```python
from build123d import *

# Parameters (mm, degrees)
BOSS_EXTRUDE2_DEPTH  = 11.1125
SKETCH1_11_W         = 50.8
SKETCH1_11_H         = 50.8
BOSS_EXTRUDE3_DEPTH  = 609.6
SKETCH1_12_W         = 50.8
SKETCH1_12_H         = 50.8
BOSS_EXTRUDE4_DEPTH  = 609.6
SKETCH1_13_W         = 50.8
SKETCH1_13_H         = 50.8
BOSS_EXTRUDE5_DEPTH  = 609.6
SKETCH1_14_W         = 50.8
SKETCH1_14_H         = 50.8
BOSS_EXTRUDE6_DEPTH  = 609.6
SKETCH4_R            = 50.8
CUT_EXTRUDE2_DEPTH   = 12.1125
SKETCH5_W            = 165.1
SKETCH5_H            = 152.4
SKETCH5_W_2          = 139.7
SKETCH5_H_2          = 127
BOSS_EXTRUDE8_DEPTH  = 17.78
SKETCH13_W           = 50.8
SKETCH13_H           = 50.8
BOSS_EXTRUDE9_DEPTH  = 381
SKETCH14_R           = 55
SKETCH14_R_2         = 50.90263009
BOSS_EXTRUDE10_DEPTH = 284.5


with BuildPart() as part:
    # Sketch1 → Boss-Extrude2 (new body)
    with BuildSketch(Plane(origin=(0, 0, 0), x_dir=(1, 0, 0), z_dir=(0, 1, 0))):
        Polygon((-136.525, 152.4), (-187.325, 152.4), (-187.325, -203.2), (187.325, -203.2), (187.325, 203.2), (-136.525, 203.2), align=None)
    extrude(amount=BOSS_EXTRUDE2_DEPTH)

    # Sketch1<11> → Boss-Extrude3 (add)
    with BuildSketch(Plane(origin=(0, 0, 0), x_dir=(1, 0, 0), z_dir=(0, 1, 0))):
        with Locations((-161.925, 177.8)):
            Rectangle(SKETCH1_11_W, SKETCH1_11_H)
    extrude(amount=BOSS_EXTRUDE3_DEPTH)

    # Sketch1<12> → Boss-Extrude4 (add)
    with BuildSketch(Plane(origin=(0, 0, 0), x_dir=(1, 0, 0), z_dir=(0, 1, 0))):
        with Locations((-161.925, -177.8)):
            Rectangle(SKETCH1_12_W, SKETCH1_12_H)
    extrude(amount=BOSS_EXTRUDE4_DEPTH)

    # Sketch1<13> → Boss-Extrude5 (add)
    with BuildSketch(Plane(origin=(0, 0, 0), x_dir=(1, 0, 0), z_dir=(0, 1, 0))):
        with Locations((161.925, 177.8)):
            Rectangle(SKETCH1_13_W, SKETCH1_13_H)
    extrude(amount=BOSS_EXTRUDE5_DEPTH)

    # Sketch1<14> → Boss-Extrude6 (add)
    with BuildSketch(Plane(origin=(0, 0, 0), x_dir=(1, 0, 0), z_dir=(0, 1, 0))):
        with Locations((161.925, -177.8)):
            Rectangle(SKETCH1_14_W, SKETCH1_14_H)
    extrude(amount=BOSS_EXTRUDE6_DEPTH)

    # Sketch4 → Cut-Extrude2 (cut, through all)
    with BuildSketch(Plane(origin=(0, 11.1125, 0), x_dir=(1, 0, 0), z_dir=(0, 1, 0))):
        Circle(SKETCH4_R)
    extrude(amount=-CUT_EXTRUDE2_DEPTH, mode=Mode.SUBTRACT)

    # Sketch5 → Boss-Extrude8 (add)
    with BuildSketch(Plane.XZ):
        Rectangle(SKETCH5_W, SKETCH5_H)
        Rectangle(SKETCH5_W_2, SKETCH5_H_2, mode=Mode.SUBTRACT)
    extrude(amount=BOSS_EXTRUDE8_DEPTH)

    # Sketch12 → Revolve-Thin1 (revolve)
    with BuildSketch(Plane.XY):
        Polygon((-63.5, -17.78), (-920.495660607, -336.662106272), (-923.982997727, -327.289887762), (-66.98733712, -8.407781489), align=None)
    revolve(axis=Axis((0, -17.78, 0), (0, -1, 0)))

    # Sketch13 → Boss-Extrude9 (add)
    with BuildSketch(Plane.XZ):
        with Locations((-161.925, 177.8)):
            Rectangle(SKETCH13_W, SKETCH13_H)
        with Locations((161.925, 177.8)):
            Rectangle(SKETCH13_W, SKETCH13_H)
        with Locations((161.925, -177.8)):
            Rectangle(SKETCH13_W, SKETCH13_H)
        with Locations((-161.925, -177.8)):
            Rectangle(SKETCH13_W, SKETCH13_H)
    extrude(amount=BOSS_EXTRUDE9_DEPTH)

    # Sketch14 → Boss-Extrude10 (add)
    with BuildSketch(Plane(origin=(0, 11.1125, 0), x_dir=(1, 0, 0), z_dir=(0, 1, 0))):
        Circle(SKETCH14_R)
        Circle(SKETCH14_R_2, mode=Mode.SUBTRACT)
    extrude(amount=BOSS_EXTRUDE10_DEPTH)


solid = part.part
```
For this review, take the finished solid that the model builds, in its own axes (mm). A direction names the side the tool comes from. Round coordinates to 2 decimals unless told otherwise and drop trailing zeros. Loops run counter-clockwise (first coordinate to the right, second up) from the corner with the lowest first, then second, coordinate; pieces in that order, holes last.
(1) Clearance check with flat-ended pins moving along their axes: P1, Ø15, axis at y = -47.5, z = -167, coming from the +X side (3 decimals); P2, Ø6, axis at x = 541, z = 174, coming from the +Y side; P3, Ø3, axis at x = -484, z = 618.5, coming from the -Y side. State where each tip first meets the part, or that it passes through.
Returned:
P1: stops at x = 187.325
P2: stops at y = -193.82
P3: stops at y = -286.94
(2) Mouldability with a two-part tool opening along Y and no side actions: class faces 1 (the flat face through (-162, -223, 152.4)), 2 (the conical face through (199.59, -336.08, 898.82)), 3 (the conical face through (63.654, -17.325, -1.4)) as released by +Y, released by -Y, zero draft, split by the parting line, or undercut.
Returned:
face 1: zero draft
face 2: released by -Y
face 3: undercut
(3) Tool access review of faces 4 (the flat face through (-136.525, -37, 177)), 5 (the flat face through (-162, -36, 152.4)), 6 (the flat face through (162, -36, 152.4)), 7 (the flat face through (-162, -223, -152.4)): name each direction out of +Z, -Z, +X, -X, +Y, -Y from which nothing blocks a thin tool from reaching the whole face with its end or side.
Returned:
face 4: +Z
face 5: -X
face 6: +X
face 7: -Y
(4) Wall thickness on line 1 along Z through (x, y) = (0, 94); line 2 along Z through (x, y) = (0, 3.5): over which ranges is each line inside the solid? List them lowest first.
Returned:
line 1: z = -55 to -50.9, 50.9 to 55
line 2: z = -203.2 to -50.8, 50.8 to 203.2
(5) We need section D-D (y = -292). Give the boundary of the cut face in (x, z) (1 decimal), plus the area to 3 significant figures.
Returned:
outline: circle Ø1658.3 at (0, 0); (-187.3, -203.2) - (-136.5, -203.2) - (-136.5, -152.4) - (-187.3, -152.4) - close; (-187.3, 152.4) - (-136.5, 152.4) - (-136.5, 203.2) - (-187.3, 203.2) - close; (136.5, -203.2) - (187.3, -203.2) - (187.3, -152.4) - (136.5, -152.4) - close; (136.5, 152.4) - (187.3, 152.4) - (187.3, 203.2) - (136.5, 203.2) - close; hole circle Ø1600.9 at (0, 0)
area: 157,000 mm2
(6) We need section A-A (y = 160). Give the boundary of the cut face in (x, z) (3 decimals), plus the area to 3 significant figures.
Returned:
outline: (-187.325, -203.2) - (-136.525, -203.2) - (-136.525, -152.4) - (-187.325, -152.4) - close; (-187.325, 152.4) - (-136.525, 152.4) - (-136.525, 203.2) - (-187.325, 203.2) - close; circle Ø110 at (0, 0); (136.525, -203.2) - (187.325, -203.2) - (187.325, -152.4) - (136.525, -152.4) - close; (136.525, 152.4) - (187.325, 152.4) - (187.325, 203.2) - (136.525, 203.2) - close; hole circle Ø101.805 at (0, 0)
area: 11,700 mm2
(7) We need section B-B (y = 442.5). Give the boundary of the cut face in (x, z) (3 decimals), plus the area to 3 significant figures.
Returned:
outline: (-187.325, -203.2) - (-136.525, -203.2) - (-136.525, -152.4) - (-187.325, -152.4) - close; (-187.325, 152.4) - (-136.525, 152.4) - (-136.525, 203.2) - (-187.325, 203.2) - close; (136.525, -203.2) - (187.325, -203.2) - (187.325, -152.4) - (136.525, -152.4) - close; (136.525, 152.4) - (187.325, 152.4) - (187.325, 203.2) - (136.525, 203.2) - close
area: 10,300 mm2
